from build123d import *

# Parameters (mm, degrees)
SKETCH1_R           = 6.1
SKETCH1_R_2         = 1.5
BOSS_EXTRUDE1_DEPTH = 2.3
SKETCH2_R           = 4.4
SKETCH2_R_2         = 3
BOSS_EXTRUDE2_DEPTH = 3.2
SKETCH3_R           = 0.75
BOSS_EXTRUDE3_DEPTH = 2.3


with BuildPart() as part:
    # Sketch1 → Boss-Extrude1 (new body)
    with BuildSketch(Plane(origin=(0, 0, 0), x_dir=(1, 0, 0), z_dir=(0, 1, 0))):
        Circle(SKETCH1_R)
        Circle(SKETCH1_R_2, mode=Mode.SUBTRACT)
    extrude(amount=BOSS_EXTRUDE1_DEPTH)

    # Sketch2 → Boss-Extrude2 (add)
    with BuildSketch(Plane(origin=(0, 2.3, 0), x_dir=(1, 0, 0), z_dir=(0, 1, 0))):
        Circle(SKETCH2_R)
        Circle(SKETCH2_R_2, mode=Mode.SUBTRACT)
    extrude(amount=BOSS_EXTRUDE2_DEPTH)

    # Sketch3 → Boss-Extrude3 (add)
    with BuildSketch(Plane.XZ):
        with BuildLine():
            Line((-4.5, -4.118252056), (-2.468988638, -16.892549493))
            ThreePointArc((-2.468988638, -16.892549493), (0, -19), (2.468988638, -16.892549493))
            Line((2.468988638, -16.892549493), (4.5, -4.118252056))
            ThreePointArc((4.5, -4.118252056), (0, -6.1), (-4.5, -4.118252056))
        make_face()
        with Locations((0, -16)):
            Circle(SKETCH3_R, mode=Mode.SUBTRACT)
        with Locations((0, -13)):
            Circle(SKETCH3_R, mode=Mode.SUBTRACT)
        with Locations((0, -10)):
            Circle(SKETCH3_R, mode=Mode.SUBTRACT)
        with Locations((0, -7)):
            Circle(SKETCH3_R, mode=Mode.SUBTRACT)
    extrude(amount=-BOSS_EXTRUDE3_DEPTH)


solid = part.part
Work out the finished part from the listing and answer in its coordinate system (mm). A direction names the side the tool comes from. Round coordinates to 2 decimals unless told otherwise and drop trailing zeros. Loops run counter-clockwise (first coordinate to the right, second up) from the corner with the lowest first, then second, coordinate; pieces in that order, holes last. Notation, with made-up numbers: (46, -2) - (81, -2) arc R25 cw to (81, 29) - close; hole circle Ø3 at (30.25, -25). An arc over 180 degrees is marked (long way). Use one line per item in the form item = value. Start each with the question number.
(1) Find section C-C on z = 0. Determine the outline of the cut face in (x, y).
(2) Determine the mould class of faces 3 (the face through (-0.197, 1.134, 6.097)), 4 (the face through (-0.098, 1.134, -9.256)), 5 (the face through (3.47, 1.13, -10.59)) for opening direction Z: +Z half, -Z half, draft (parallel to the pull), parting line (faces both ways), or undercut.
(3) Find section B-B on y = 1.3. Determine the outline of the cut face in (x, z).
(4) Flat-ended cylindrical pins translate along their axes: P1, Ø3, axis at x = 0, z = -1, coming from the +Y side; P2, Ø1, axis at x = 0.5, y = 3, coming from the +Z side; P3, Ø3, axis at x = 2, y = 3, coming from the +Z side; P4, Ø0.9, axis at x = 0, z = -7, coming from the +Y side. Find the tip coordinate at first contact, or state that the pin passes through.
(5) Which of the six approach directions +Z, -Z, +X, -X, +Y, -Y give full straight-line access (tool end or side, diameter ignored) to faces 1 (the face through (-1.5, 1.13, -0.07)), 2 (the face through (-3, 4, 0))?
(6) Consider line 1 (Z direction, x = 0, y = 1.7); line 2 (X direction, y = 1.1, z = 0); line 3 (X direction, y = 3.9, z = 0). Determine where each line is inside the solid, lowest interval first.
(7) Find section A-A on x = 0. Give the number of separate pieces and of enclosed holes in the cut face, and give its area (3 significant figures).
(8) Find section D-D on z = -13. Determine the outline of the cut face in (x, y), and give its area (3 significant figures).
Answer list:
q1.outline = (-6.1, 0) - (-1.5, 0) - (-1.5, 2.3) - (-3, 2.3) - (-3, 5.5) - (-4.4, 5.5) - (-4.4, 2.3) - (-6.1, 2.3) - close; (1.5, 0) - (6.1, 0) - (6.1, 2.3) - (4.4, 2.3) - (4.4, 5.5) - (3, 5.5) - (3, 2.3) - (1.5, 2.3) - close
q2.face_3 = parting line
q2.face_4 = undercut
q2.face_5 = -Z half
q3.outline = (-4.5, -4.12) - (-2.47, -16.89) arc R2.5 ccw to (2.47, -16.89) - (4.5, -4.12) arc R6.1 ccw (long way) to start; hole circle Ø3 at (0, 0); hole circle Ø1.5 at (0, -16); hole circle Ø1.5 at (0, -13); hole circle Ø1.5 at (0, -10); hole circle Ø1.5 at (0, -7)
q4.P1 = 2.3
q4.P2 = 4.4
q4.P3 = 6.06
q4.P4 = through
q5.face_1 = +Y, -Y
q5.face_2 = +Y
q6.line_1 = -19 to -16.75, -15.25 to -13.75, -12.25 to -10.75, -9.25 to -7.75, -6.25 to -1.5, 1.5 to 6.1
q6.line_2 = -6.1 to -1.5, 1.5 to 6.1
q6.line_3 = -4.4 to -3, 3 to 4.4
q7.separate_pieces = 6
q7.enclosed_holes = 0
q7.area = 46.0 mm^2
q8.outline = (-3.09, 0) - (-0.75, 0) - (-0.75, 2.3) - (-3.09, 2.3) - close; (0.75, 0) - (3.09, 0) - (3.09, 2.3) - (0.75, 2.3) - close
q8.area = 10.8 mm^2
